```python
from build123d import *

# Parameters (mm, degrees)
SKETCH1_R           = 13
SKETCH1_R_2         = 2.75
BOSS_EXTRUDE1_DEPTH = 3
BOSS_EXTRUDE2_START = -3
BOSS_EXTRUDE2_DEPTH = 3
FILLET1_R           = 0.5
CIRPATTERN1_COUNT   = 4
CIRPATTERN1_ANGLE   = 60
CIRPATTERN2_COUNT   = 4
CIRPATTERN2_ANGLE   = 60
SKETCH3_R           = 2.125
BOSS_EXTRUDE3_DEPTH = 3
FILLET2_R           = 0.5


with BuildPart() as part:
    # Sketch1 → Boss-Extrude1 (new body)
    with BuildSketch(Plane.XY):
        with Locations((43.95, -5.65)):
            Circle(SKETCH1_R)
        with Locations((43.95, -5.65)):
            Circle(SKETCH1_R_2, mode=Mode.SUBTRACT)
    extrude(amount=BOSS_EXTRUDE1_DEPTH)

    # Sketch2 → Boss-Extrude2 (add)
    with BuildSketch(Plane.XY.offset(3).offset(BOSS_EXTRUDE2_START)):
        with BuildLine():
            Line((27.95, -4.9), (27.95, -6.4))
            ThreePointArc((27.95, -6.4), (29.455813765, -6.929754851), (31.03682843, -7.15))
            ThreePointArc((31.03682843, -7.15), (30.95, -5.65), (31.03682843, -4.15))
            ThreePointArc((31.03682843, -4.15), (29.455813765, -4.370245149), (27.95, -4.9))
        make_face()
    boss_extrude2 = extrude(amount=BOSS_EXTRUDE2_DEPTH)

    # Fillet1
    fillet1_edges = [part.edges().sort_by_distance(p)[0] for p in [
        (31.03682843, -7.15, 1.5),
        (27.95, -6.4, 1.5),
        (27.95, -4.9, 1.5),
        (31.03682843, -4.15, 1.5),
    ]]
    fillet(fillet1_edges, radius=FILLET1_R)

    # CirPattern1: Boss-Extrude2 ×4 about axis
    cirpattern1_axis = Axis((43.95, -5.65, 0), (0, 0, -1))
    for i in range(1, CIRPATTERN1_COUNT):
        add(boss_extrude2.rotate(cirpattern1_axis, i * CIRPATTERN1_ANGLE / (CIRPATTERN1_COUNT - 1)))

    # CirPattern2: Boss-Extrude2 ×4 about axis
    cirpattern2_axis = Axis((43.95, -5.65, 0), (0, 0, 1))
    for i in range(1, CIRPATTERN2_COUNT):
        add(boss_extrude2.rotate(cirpattern2_axis, i * CIRPATTERN2_ANGLE / (CIRPATTERN2_COUNT - 1)))

    # Sketch3 → Boss-Extrude3 (add)
    with BuildSketch(Plane.XY.offset(3)):
        with BuildLine():
            Line((43.799969992, 1.109522125), (57.880684913, 21.218867074))
            ThreePointArc((57.880684913, 21.218867074), (63.451598836, 22.201169506), (64.433901268, 16.630255583))
            Line((64.433901268, 16.630255583), (49.86779594, -4.172298707))
            Line((49.86779594, -4.172298707), (43.799969992, 1.109522125))
        make_face()
        with Locations((61.157293091, 18.924561329)):
            Circle(SKETCH3_R, mode=Mode.SUBTRACT)
    extrude(amount=-BOSS_EXTRUDE3_DEPTH)

    # Fillet2
    fillet2_edges = [part.edges().sort_by_distance(p)[0] for p in [
        (36.599519053, -19.881406461, 1.5),
        (35.300480947, -19.131406461, 1.5),
        (28.65840296, -0.882447172, 1.5),
        (29.171433175, 0.527091759, 1.5),
        (31.211198203, 4.060068423, 1.5),
        (32.175379617, 5.209135087, 1.5),
        (35.300480947, 7.831406461, 1.5),
        (36.599519053, 8.581406461, 1.5),
        (29.171433175, -11.827091759, 1.5),
        (28.65840296, -10.417552828, 1.5),
        (32.175379617, -16.509135087, 1.5),
        (31.211198203, -15.360068423, 1.5),
    ]]
    fillet(fillet2_edges, radius=FILLET2_R)


solid = part.part
```
Work out the finished part from the listing and answer in its coordinate system (mm). A direction names the side the tool comes from. Give positions to 0.01 mm unless a question says otherwise; leave off trailing zeros. Loops run counter-clockwise (first coordinate to the right, second up) from the corner with the lowest first, then second, coordinate; pieces in that order, holes last. Notation, with made-up numbers: (-28.75, -20) -> (-5.75, -20) arc R13 ccw to (-5.75, -1) -> close; hole circle Ø2 at (71, -36.5). An arc over 180 degrees is marked (long way). One line per question, with ' | ' between items. Start each with the question number.
1) Section A-A, the plane x = 43.95 is taken. Determine the outline of the cut face in (y, z).
2) Section D-D, the plane y = -14.5 is taken. Determine the outline of the cut face in (x, z).
3) Each of these flat-tipped pins is pushed along its axis until it touches: pin 1 (1.5 mm diameter, centred on y = 1, z = 2, fed in from +X); pin 2 (1 mm diameter, centred on x = 47.5, z = 0.5, fed in from -Y); pin 3 (1.5 mm diameter, centred on x = 32.5, z = 1, fed in from -Y). Where does it stop, or does it pass through?
4) Section C-C, the plane z = 1.9 is taken. State how many separate pieces and enclosed holes the cut face has, then the cut area to 3 significant figures.
5) Section B-B, the plane x = 55 is taken. Determine the outline of the cut face in (y, z).
6) Straight lines are drawn through the part: L1, parallel to Y at x = 43.95, z = 0.7; L2, parallel to Y at x = 42, z = 1; L3, parallel to Y at x = 32.5, z = 2.4. For each, find the intervals that lie inside material, in ascending order.
7) Determine the mould class of faces 1 (the face through (30.05, -9.3, 1.48)), 2 (the face through (33.84, 4.56, 1.48)), 3 (the face through (46, -3, 0)) for opening direction X: +X half, -X half, draft (parallel to the pull), parting line (faces both ways), or undercut.
8) For faces 4 (the face through (59.45, 9.51, 1.52)), 5 (the face through (30.954, 0.487, 1.479)), 6 (the face through (32.137, -13.836, 1.479)), 7 (the face through (37.912, -18.734, 1.479)), determine the directions among +Z, -Z, +X, -X, +Y, -Y from which every point of the face is accessible in a straight line to the end or side of a thin tool.
Resolved:
1) outline: (-18.65, 0) -> (-8.4, 0) -> (-8.4, 3) -> (-18.65, 3) -> close; (-2.9, 0) -> (7.35, 0) -> (7.35, 3) -> (-2.9, 3) -> close
2) outline: (31.68, 0) -> (53.47, 0) -> (53.47, 3) -> (31.68, 3) -> close
3) pin 1: x = 55.53 | pin 2: y = -18.29 | pin 3: y = -16.44
4) separate pieces: 1 | enclosed holes: 2 | area: 708 mm2
5) outline: (-12.5, 0) -> (1.2, 0) -> (1.2, 3) -> (-12.5, 3) -> close; (3.16, 0) -> (17.1, 0) -> (17.1, 3) -> (3.16, 3) -> close
6) L1: -18.65 to -8.4, -2.9 to 7.35 | L2: -18.5 to -7.59, -3.71 to 7.2 | L3: -16.42 to -13.4, -11.81 to 0.51, 2.1 to 5.12
7) face 1: -X half | face 2: undercut | face 3: draft
8) face 4: +Z, -Z, +X | face 5: +Z, -Z | face 6: +Z, -Z, -X | face 7: +Z, -Z, -Y
